Model file for the job. Use its own axes, mm. A direction names the side the tool comes from. Round coordinates to 2 decimals unless told otherwise and drop trailing zeros. Order: outer loops, then holes, each group sorted by start corner. A loop starts at its lowest first (then second) coordinate and runs counter-clockwise, first axis right, second up. Notation, with made-up numbers: (-8.75, 83.5) -> (-4.75, 83.5) arc R21 ccw to (-4.75, 118.5) -> close; hole circle Ø8 at (53, 24.25). An arc over 180 degrees is marked (long way). Put each result on its own line as item: value. Start each with the question number.
Q1. Cut at A-A, the plane z = 40. List the corners of the cut face in (x, y), and give its area (3 significant figures).
Q2. Cut at B-B, the plane z = 33.5. List the corners of the cut face in (x, y).
Q3. Cut at C-C, the plane x = 7. State how many separate pieces and enclosed holes the cut face has, and give its area (3 significant figures).
Q4. Pull direction X, two halves, no side cores. Call faces 5 (the face through (0, -6, 10)), 6 (the face through (4.315, 4.463, 15.135)), 7 (the face through (-4.58, 4.24, 15.14)), 8 (the face through (-1.172, 8.923, 17.986)): released by +X, released by -X, zero draft, split by the parting line, or undercut.
Q5. Flat gauge pins, fed straight in: P1, Ø1, axis at x = 0, y = -7, coming from the -Z side; P2, Ø0.6, axis at x = 5, z = 41.5, coming from the -Y side; P3, Ø8, axis at y = -4.5, z = 21.5, coming from the -X side. Where does each tip first touch, or does it go through?
Q6. Probe L1, parallel to Y at x = 0, z = 14; L2, parallel to Y at x = 0, z = 34.5; L3, parallel to X at y = -7, z = 15.5. List the from-to ranges inside material, lowest first.
Q7. 3-axis set-ups, long thin cutter, end or side, ignore diameter. For faces 1 (the face through (-3.86, 3.92, 41.46)), 2 (the face through (-3.92, -3.86, 41.46)), 3 (the face through (-0.104, -6.207, 15.135)), 4 (the face through (3.92, 3.86, 41.46)): which of +Z, -Z, +X, -X, +Y, -Y reach the whole face in a straight line?
from build123d import *

# Parameters (mm, degrees)
ESQUISSE1_R                                   = 5.5
ESQUISSE1_R_2                                 = 4.5
BOSS_EXTRU_1_DEPTH                            = 10
ESQUISSE3_R                                   = 8.5
ESQUISSE3_R_2                                 = 5
BOSS_EXTRU_3_DEPTH                            = 7
ESQUISSE4_R                                   = 9
ESQUISSE4_R_2                                 = 5
BOSS_EXTRU_4_DEPTH                            = 2
ESQUISSE7_R                                   = 6
ESQUISSE7_R_2                                 = 5
BOSS_EXTRU_7_DEPTH                            = 11
ESQUISSE8_R                                   = 9
ESQUISSE8_R_2                                 = 5
BOSS_EXTRU_8_DEPTH                            = 2
ESQUISSE15_R                                  = 8.5
ESQUISSE15_R_2                                = 5
BOSS_EXTRU_9_DEPTH                            = 7
ESQUISSE16_R                                  = 5.5
ESQUISSE16_R_2                                = 5
BOSS_EXTRU_10_DEPTH                           = 5
ESQUISSE17_W                                  = 20
ESQUISSE17_H                                  = 2
ESQUISSE17_W_2                                = 2
ESQUISSE17_H_2                                = 20
ENL_V_MAT_EXTRU_1_DEPTH                       = 5
TROU_POUR_TARAUDAGE_POUR_TROU_TARAUD_M2_D     = 1.6
TROU_POUR_TARAUDAGE_POUR_TROU_TARAUD_M2_DEPTH = 9
CONG_1_R                                      = 2


with BuildPart() as part:
    # Esquisse1 → Boss.-Extru.1 (new body)
    with BuildSketch(Plane.XY):
        Circle(ESQUISSE1_R)
        Circle(ESQUISSE1_R_2, mode=Mode.SUBTRACT)
    extrude(amount=BOSS_EXTRU_1_DEPTH)

    # Esquisse3 → Boss.-Extru.3 (add)
    with BuildSketch(Plane.XY.offset(10)):
        Circle(ESQUISSE3_R)
        Circle(ESQUISSE3_R_2, mode=Mode.SUBTRACT)
    extrude(amount=BOSS_EXTRU_3_DEPTH)

    # Esquisse4 → Boss.-Extru.4 (add)
    with BuildSketch(Plane.XY.offset(17)):
        Circle(ESQUISSE4_R)
        Circle(ESQUISSE4_R_2, mode=Mode.SUBTRACT)
    extrude(amount=BOSS_EXTRU_4_DEPTH)

    # Esquisse7 → Boss.-Extru.7 (add)
    with BuildSketch(Plane.XY.offset(19)):
        Circle(ESQUISSE7_R)
        Circle(ESQUISSE7_R_2, mode=Mode.SUBTRACT)
    extrude(amount=BOSS_EXTRU_7_DEPTH)

    # Esquisse8 → Boss.-Extru.8 (add)
    with BuildSketch(Plane.XY.offset(30)):
        Circle(ESQUISSE8_R)
        Circle(ESQUISSE8_R_2, mode=Mode.SUBTRACT)
    extrude(amount=BOSS_EXTRU_8_DEPTH)

    # Esquisse15 → Boss.-Extru.9 (add)
    with BuildSketch(Plane.XY.offset(32)):
        Circle(ESQUISSE15_R)
        Circle(ESQUISSE15_R_2, mode=Mode.SUBTRACT)
    extrude(amount=BOSS_EXTRU_9_DEPTH)

    # Esquisse16 → Boss.-Extru.10 (add)
    with BuildSketch(Plane.XY.offset(39)):
        Circle(ESQUISSE16_R)
        Circle(ESQUISSE16_R_2, mode=Mode.SUBTRACT)
    extrude(amount=BOSS_EXTRU_10_DEPTH)

    # Esquisse17 → Enlèv. mat.-Extru.1 (cut)
    with BuildSketch(Plane.XY.offset(44)):
        Rectangle(ESQUISSE17_W, ESQUISSE17_H)
        Rectangle(ESQUISSE17_W_2, ESQUISSE17_H_2)
    extrude(amount=-ENL_V_MAT_EXTRU_1_DEPTH, mode=Mode.SUBTRACT)

    # Trou pour taraudage pour trou taraudé M21
    with Locations(Plane(origin=(0, 0, 10), x_dir=(-1, 0, 0), z_dir=(0, 0, -1))):
        with Locations((-7, 0), (-4.949747468, 4.949747468), (0, 7), (4.949747468, 4.949747468), (7, 0), (4.949747468, -4.949747468), (0, -7), (-4.949747468, -4.949747468), (0, 0)):
            Hole(TROU_POUR_TARAUDAGE_POUR_TROU_TARAUD_M2_D / 2, depth=TROU_POUR_TARAUDAGE_POUR_TROU_TARAUD_M2_DEPTH)

    # Congé1
    # the kernel refuses this fillet: 2 mm, written as the material it adds along each edge
    with BuildSketch(Plane(origin=(0, 0, 30), x_dir=(1, 0, 0), z_dir=(0, -1, 0))) as cong_1_piece_1:
        with BuildLine():
            CenterArc((6 + CONG_1_R, -CONG_1_R), CONG_1_R, 90, 90)
            Line((6 + CONG_1_R, 0), (6, 0))
            Line((6, 0), (6, -CONG_1_R))
        make_face()
    revolve(axis=Axis((0, 0, 30), (0, 0, 1)))
    with BuildSketch(Plane(origin=(0, 0, 19), x_dir=(1, 0, 0), z_dir=(0, -1, 0))) as cong_1_piece_2_section:
        with BuildLine():
            CenterArc((6 + CONG_1_R, CONG_1_R), CONG_1_R, 180, 90)
            Line((6, CONG_1_R), (6, 0))
            Line((6, 0), (6 + CONG_1_R, 0))
        make_face()
    cong_1_piece_2 = revolve(axis=Axis((0, 0, 19), (0, 0, 1)), mode=Mode.PRIVATE)
    cong_1_piece_2 = cong_1_piece_2 - Plane(origin=(-4.949747468, -4.949747468, 19.036420824), x_dir=(1, 0, 0), z_dir=(0, 0, 1)) * Cylinder(0.8, 32, mode=Mode.PRIVATE)
    cong_1_piece_2 = cong_1_piece_2 - Plane(origin=(0, -7, 19.036420824), x_dir=(1, 0, 0), z_dir=(0, 0, 1)) * Cylinder(0.8, 32, mode=Mode.PRIVATE)
    cong_1_piece_2 = cong_1_piece_2 - Plane(origin=(4.949747468, -4.949747468, 19.036420824), x_dir=(1, 0, 0), z_dir=(0, 0, 1)) * Cylinder(0.8, 32, mode=Mode.PRIVATE)
    cong_1_piece_2 = cong_1_piece_2 - Plane(origin=(-7, 0, 19.036420824), x_dir=(1, 0, 0), z_dir=(0, 0, 1)) * Cylinder(0.8, 32, mode=Mode.PRIVATE)
    cong_1_piece_2 = cong_1_piece_2 - Plane(origin=(-4.949747468, 4.949747468, 19.036420824), x_dir=(1, 0, 0), z_dir=(0, 0, 1)) * Cylinder(0.8, 32, mode=Mode.PRIVATE)
    cong_1_piece_2 = cong_1_piece_2 - Plane(origin=(7, 0, 19.036420824), x_dir=(1, 0, 0), z_dir=(0, 0, 1)) * Cylinder(0.8, 32, mode=Mode.PRIVATE)
    cong_1_piece_2 = cong_1_piece_2 - Plane(origin=(0, 7, 19.036420824), x_dir=(1, 0, 0), z_dir=(0, 0, 1)) * Cylinder(0.8, 32, mode=Mode.PRIVATE)
    cong_1_piece_2 = cong_1_piece_2 - Plane(origin=(4.949747468, 4.949747468, 19.036420824), x_dir=(1, 0, 0), z_dir=(0, 0, 1)) * Cylinder(0.8, 32, mode=Mode.PRIVATE)
    add(cong_1_piece_2)


solid = part.part
Ans:
1. outline: (-5.41, -1) arc R5.5 ccw to (-1, -5.41) -> (-1, -4.9) arc R5 cw to (-4.9, -1) -> close; (-5.41, 1) -> (-4.9, 1) arc R5 cw to (-1, 4.9) -> (-1, 5.41) arc R5.5 ccw to start; (1, -5.41) arc R5.5 ccw to (5.41, -1) -> (4.9, -1) arc R5 cw to (1, -4.9) -> close; (1, 4.9) arc R5 cw to (4.9, 1) -> (5.41, 1) arc R5.5 ccw to (1, 5.41) -> close
1. area: 12.5 mm^2
2. outline: circle Ø17 at (0, 0); hole circle Ø10 at (0, 0)
3. separate pieces: 3
3. enclosed holes: 0
3. area: 168 mm^2
4. face 5: zero draft
4. face 6: undercut
4. face 7: undercut
4. face 8: split by the parting line
5. P1: stops at z = 29.32
5. P2: stops at y = -2.86
5. P3: stops at x = -8.89
6. L1: y = -8.5 to -7.8, -6.2 to -5, 5 to 6.2, 7.8 to 8.5
6. L2: y = -8.5 to -5, 5 to 8.5
6. L3: x = -4.82 to -0.8, 0.8 to 4.82
7. face 1: +Z, -X, +Y
7. face 2: +Z, -X, -Y
7. face 3: -Z
7. face 4: +Z, +X, +Y
